Model file for the job. Use its own axes, mm. A direction names the side the tool comes from. Coordinates: 2 decimals unless noted, no trailing zeros. Order: outer loops, then holes, each group sorted by start corner. A loop starts at its lowest first (then second) coordinate and runs counter-clockwise, first axis right, second up. Notation, with made-up numbers: (71.25, 62.25) -> (130.25, 62.25) arc R28 cw to (130.25, 88.25) -> close; hole circle Ø3 at (88, -17). An arc over 180 degrees is marked (long way). Use CSV: the item, a comma, the result in double quotes. Start each with the question number.
(1) Pin check, flat tips, straight feed: pin 1 Ø1.3 at (x, y) = (-2, -1) entering from -Z; pin 2 Ø0.6 at (y, z) = (-0.5, -16) entering from +X; pin 3 Ø0.7 at (x, z) = (-0.5, -14.5) entering from +Y. Stop position of each tip, or through.
(2) Probe L1, parallel to Z at x = 9, y = -0.4. List the from-to ranges inside material, lowest first.
(3) Cut at A-A on y = -0.4. Write the cut outline in (x, z), plus the area to 3 significant figures.
(4) Cut at B-B on x = 2.5. Write the cut outline in (y, z).
(5) Tool access for faces 1 (the flat face through (0, -2.54, 0)), 2 (the flat face through (0, -1.269, -15)): list every direction of +Z, -Z, +X, -X, +Y, -Y with a clear straight run to the whole face (end or side of a thin tool).
(6) Cut at C-C on y = -1.85. Write the cut outline in (x, z).
```python
from build123d import *

# Parameters (mm, degrees)
F0_W     = 25.1511335373
F0_H     = 26.5552401543
F1_DEPTH = 2.54
F2_W     = 2.3688124493
F2_H     = 0.4084529355
F3_DEPTH = 2.8681720141
F4_W     = 0.3632875159
F4_H     = 0.8602547459
F5_DEPTH = 0.7417961024


with BuildPart() as f1:
    # F0 (on Front) → F1 (new body)
    with BuildSketch(Plane.XZ):
        Rectangle(F0_W, F0_H)
    extrude(amount=F1_DEPTH)

    # F2 (on face) → F3 (join)
    with BuildSketch(Plane(origin=(0, 0, -13.2776200771), x_dir=(1, 0, 0), z_dir=(0, 0, -1))):
        with Locations((0, 1.0644812137)):
            Rectangle(F2_W, F2_H)
    extrude(amount=F3_DEPTH)

    # F4 (on face) → F5 (join)
    with BuildSketch(Plane(origin=(0, 0, -16.1457920913), x_dir=(1, 0, 0), z_dir=(0, 0, -1))):
        with Locations((-0.0494890846, 0.430127373)):
            Rectangle(F4_W, F4_H)
    extrude(amount=-F5_DEPTH)


solid = f1.part
```
Outcome:
1,pin 1,"z = -13.28"
1,pin 2,"x = 0.13"
1,pin 3,"y = -0.86"
2,L1,"-13.28 to 13.28"
3,outline,"(-12.58, -13.28) -> (12.58, -13.28) -> (12.58, 13.28) -> (-12.58, 13.28) -> close; (-0.23, -16.15) -> (0.13, -16.15) -> (0.13, -15.4) -> (-0.23, -15.4) -> close"
3,area,"668 mm2"
4,outline,"(-2.54, -13.28) -> (0, -13.28) -> (0, 13.28) -> (-2.54, 13.28) -> close"
5,face 1,"+Z, -Z, +X, -X, -Y"
5,face 2,"-Z, +X, -X, -Y"
6,outline,"(-12.58, -13.28) -> (12.58, -13.28) -> (12.58, 13.28) -> (-12.58, 13.28) -> close"
